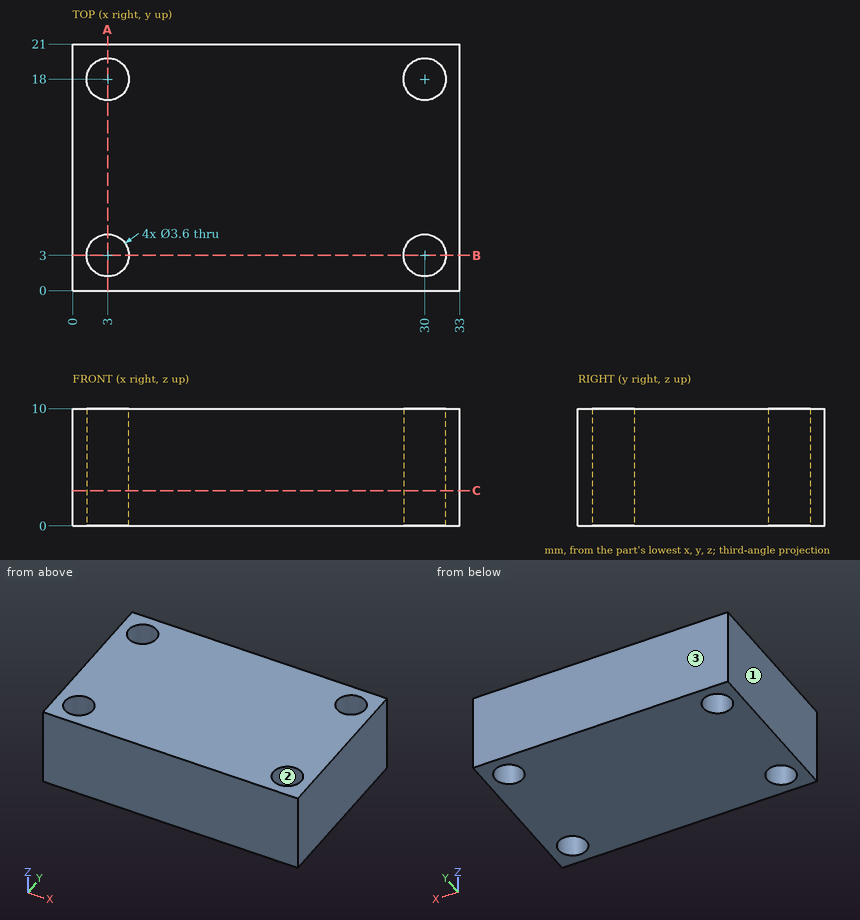
Design review of the part shown in the three views and the two pictorial views. Dimensions are in mm from the part's minimum x, y and z. Give positions to 0.01 mm unless a question says otherwise; leave off trailing zeros. Loops run counter-clockwise (first coordinate to the right, second up) from the corner with the lowest first, then second, coordinate; pieces in that order, holes last. Notation, with made-up numbers: (39.5, 80) -> (69.5, 80) arc R8 cw to (69.5, 95) -> close; hole circle Ø11 at (46, 3). An arc over 180 degrees is marked (long way). Answer as a JSON object with one key per item and string values. Group by question number.
Q1. Draft analysis for pull direction X (two halves, no side actions). For the marked faces 1, 2 and 3, state which applies: pulls with the +X half, pulls with the -X half, needs draft (parallel to the pull), parting line crosses it, or undercut.
Q2. Take a section at A-A (x = 3). Write out the cut boundary in (y, z).
Q3. Take a section at C-C (z = 3). Write out the cut boundary in (x, y).
Q4. Take a section at B-B (y = 3). Write out the cut boundary in (x, z).
Q5. Insertion check: pin 1 (2 mm diameter, centred on x = 30, y = 18, fed in from -Z). The pin has a flat end and moves straight along its axis. Give the tip position at first contact, or say it passes through.
Q6. Wall thickness on line 1 along X through (y, z) = (3, 4.25); line 2 along Y through (x, z) = (3, 6.25); line 3 along X through (y, z) = (17, 9.5): over which ranges is each line inside the solid? List them lowest first.
Answer below:
{
 "1": {"face 1": "pulls with the -X half", "face 2": "undercut", "face 3": "needs draft"},
 "2": {"outline": "(0, 0) -> (1.2, 0) -> (1.2, 10) -> (0, 10) -> close; (4.8, 0) -> (16.2, 0) -> (16.2, 10) -> (4.8, 10) -> close; (19.8, 0) -> (21, 0) -> (21, 10) -> (19.8, 10) -> close"},
 "3": {"outline": "(0, 0) -> (33, 0) -> (33, 21) -> (0, 21) -> close; hole circle Ø3.6 at (3, 3); hole circle Ø3.6 at (3, 18); hole circle Ø3.6 at (30, 3); hole circle Ø3.6 at (30, 18)"},
 "4": {"outline": "(0, 0) -> (1.2, 0) -> (1.2, 10) -> (0, 10) -> close; (4.8, 0) -> (28.2, 0) -> (28.2, 10) -> (4.8, 10) -> close; (31.8, 0) -> (33, 0) -> (33, 10) -> (31.8, 10) -> close"},
 "5": {"pin 1": "passes through"},
 "6": {"line 1": "x = 0 to 1.2, 4.8 to 28.2, 31.8 to 33", "line 2": "y = 0 to 1.2, 4.8 to 16.2, 19.8 to 21", "line 3": "x = 0 to 1.5, 4.5 to 28.5, 31.5 to 33"}
}
